Autodesk Inventor part; units mm, degrees
ref_plane "YZ Plane" through (0, 0, 0) normal (1, 0, 0) x (0, 1, 0)
ref_plane "XZ Plane" through (0, 0, 0) normal (0, 1, 0) x (-1, 0, 0)
ref_plane "XY Plane" through (0, 0, 0) normal (0, 0, 1) x (1, 0, 0)
sketch "Sketch1" plane through (0, 0, 0) normal (0, 0, 1) x (1, 0, 0)
  line L0 (0, 0) -> (0, 25)
  line L1 (0, 25) -> (18, 25)
  line L2 (18, 25) -> (18, 22)
  line L3 (18, 22) -> (3, 22)
  line L4 (3, 22) -> (3, 0)
  line L5 (3, 0) -> (0, 0)
  dimension "d0" = 25
  dimension "d1" = 3
  dimension "d2" = 3
  dimension "d3" = 15
extrude "Extrusion1" add sketch "Sketch1" along normal blind 14
fillet "Fillet1" radius 7 2 edges at (1.5, 0, 14) (1.5, 0, 0)
sketch "Sketch2" plane through (3, 22, 14) normal (1, 0, 0) x (0, 0, -1)
  line L0 (14, 3) -> (0, 3)
  line L1 (0, -15) -> (0, 0)
  arc A0 (0, -15) -> (14, -15) centre (7, -15) ccw
  line L2 (14, -15) -> (14, 0)
  line L3 (14, 0) -> (0, 0)
  line L4 (0, -15) -> (0, 0)
  point P0 (14, -22)
  point P1 (7, -15)
  dimension "d7" = 18
  dimension "d8" = 7
hole "Hole1" at (3, 7, 7) direction (-1, 0, 0) diameter 6.647 end through all
sketch "Sketch3" plane through (0, 25, 0) normal (0, 1, 0) x (1, 0, 0)
  line L0 (18, -14) -> (0, -14)
  line L1 (0, 0) -> (0, -14)
  point P0 (10, -10.5)
  point P1 (10, -3.5)
  dimension "d16" = 7
  dimension "d17" = 3.5
  dimension "d18" = 10
  dimension "d19" = 10
hole "Hole2" at (10, 25, 10.5) at (10, 25, 3.5) direction (0, -1, 0) diameter 3 end through all
fillet "Fillet2" radius 3 2 edges at (18, 23.5, 0) (18, 23.5, 14)
properties part number "HUDSON-1-77"
Geometry: final body of the model. Coordinates: model frame, mm. A direction names the side the tool comes from. Coordinates: 2 decimals unless noted, no trailing zeros. Write each loop counter-clockwise with the first axis right and the second up, starting at its lowest first coordinate (ties: lowest second). Pieces come first, ordered by that corner, then holes. Notation, with made-up numbers: (30, 37.25) - (76, 37.25) arc R17 cw to (76, 51.25) - close; hole circle Ø4 at (86.25, -2.5). An arc over 180 degrees is marked (long way). Return JSON: item names as keys, results as strings.
Item 1: Pull-direction query (Y, two-part tool) for faces 3 (the face through (1.48, 8.27, 3.93)), 4 (the face through (1.5, 2, 11.9)), 5 (the face through (10.9, 23.5, 9.3)); classes: +Y half, -Y half, draft (parallel to the pull), parting line (faces both ways), or undercut.
Completed:
{"face 3": "undercut", "face 4": "-Y half", "face 5": "draft"}
Item 2: Line query: L1, parallel to Z at x = 10, y = 23.6; L2, parallel to Z at x = 0.7, y = 7; L3, parallel to X at y = 23.05, z = 3.5. Output: solid intervals per line, ascending.
Completed:
{"L1": "z = 0 to 2, 5 to 9, 12 to 14", "L2": "z = 0 to 3.68, 10.32 to 14", "L3": "x = 0 to 8.5, 11.5 to 18"}
Item 3: Section query B-B (x = 12.5). Output: boundary loops of the cut face in (y, z).
Completed:
{"outline": "(22, 0) - (25, 0) - (25, 14) - (22, 14) - close"}
Item 4: Section query A-A (y = 5.5). Output: boundary loops of the cut face in (x, z), and give its area (3 significant figures).
Completed:
{"outline": "(0, 0.16) - (3, 0.16) - (3, 4.03) - (0, 4.03) - close; (0, 9.97) - (3, 9.97) - (3, 13.84) - (0, 13.84) - close", "area": "23.2 mm2"}
Item 5: Pin query (flat end, axial travel): pin 1 Ø1 at (x, z) = (9, 11) entering from -Y; pin 2 Ø1.5 at (y, z) = (19, 6) entering from +X. Return the tip coordinate at first contact, or that it passes through.
Completed:
{"pin 1": "stops at y = 22", "pin 2": "stops at x = 3"}
Item 6: Section query C-C (y = 18.75). Output: boundary loops of the cut face in (x, z), and give its area (3 significant figures).
Completed:
{"outline": "(0, 0) - (3, 0) - (3, 14) - (0, 14) - close", "area": "42.0 mm2"}
Item 7: Reachability of faces 1 (the face through (18, 24, 7)), 2 (the face through (11, 22, 7)) from +Z, -Z, +X, -X, +Y, -Y: full face, straight path, thin tool, end or side. Return the list, or none.
Completed:
{"face 1": "+Z, -Z, +X, +Y, -Y", "face 2": "+Z, -Z, +X, -Y"}
